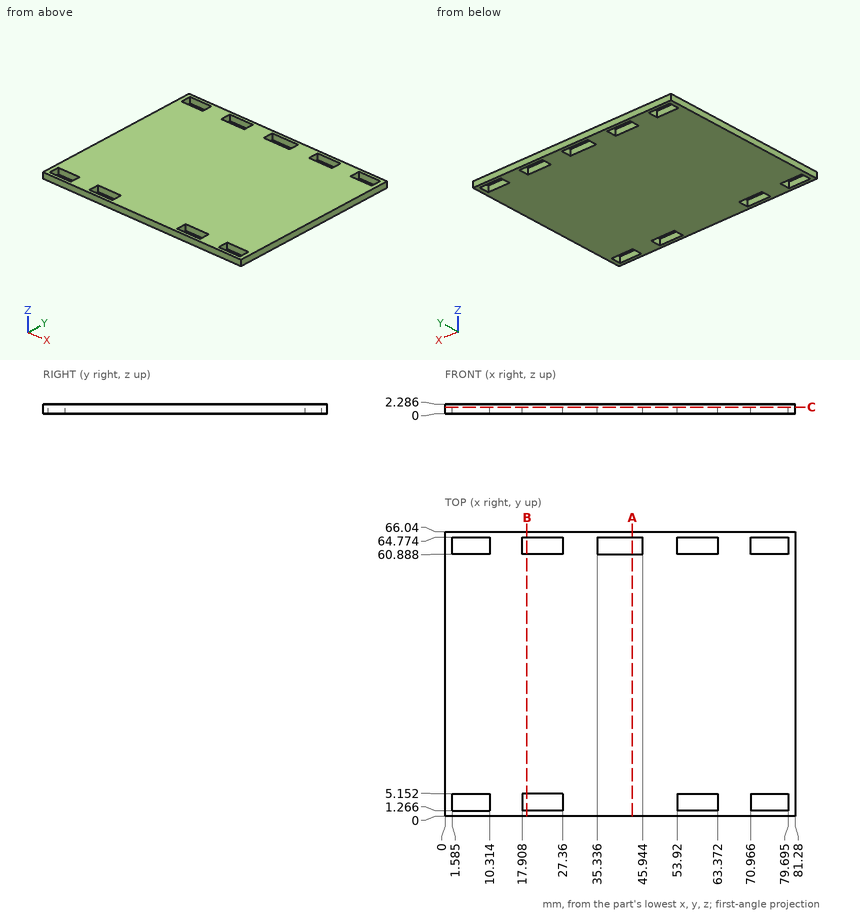
Input: dimensioned drawing with shaded views. Units: mm. Origin: part minimum x, y, z. Round coordinates to 2 decimals unless told otherwise and drop trailing zeros. Order: outer loops, then holes, each group sorted by start corner. A loop starts at its lowest first (then second) coordinate and runs counter-clockwise, first axis right, second up.
1. Material intervals for line 1 (Y direction, x = 24.5, z = 0.9) (1 decimal), sorted ascending.
The answers:
line 1: y = 0 to 1.3, 5.2 to 60.9, 64.8 to 66
2. Cut plane A-A, the plane x = 43.5. Output: boundary loops of the cut face in (y, z) (1 decimal), then the cut area to 3 significant figures.
The answers:
outline: (0, 0) - (60.9, 0) - (60.9, 2.3) - (0, 2.3) - close; (64.8, 0) - (66, 0) - (66, 2.3) - (64.8, 2.3) - close
area: 142 mm2
3. Cut plane C-C, the plane z = 1.55. State how many separate pieces and enclosed holes the cut face has, then the cut area to 3 significant figures.
The answers:
separate pieces: 1
enclosed holes: 9
area: 5,040 mm2
4. Cut plane B-B, the plane x = 19. Output: boundary loops of the cut face in (y, z) (1 decimal).
The answers:
outline: (0, 0) - (1.3, 0) - (1.3, 2.3) - (0, 2.3) - close; (5.2, 0) - (60.9, 0) - (60.9, 2.3) - (5.2, 2.3) - close; (64.8, 0) - (66, 0) - (66, 2.3) - (64.8, 2.3) - close
